Design review of the part built by this model. Coordinates are the model's own, in mm. A direction names the side the tool comes from. Round coordinates to 2 decimals unless told otherwise and drop trailing zeros. Order: outer loops, then holes, each group sorted by start corner. A loop starts at its lowest first (then second) coordinate and runs counter-clockwise, first axis right, second up. Notation, with made-up numbers: (-32, 60) - (15, 60) arc R25 cw to (15, 92) - close; hole circle Ø10 at (75.5, 88). An arc over 180 degrees is marked (long way). Use CSV: the item, a comma, the result in double quotes.
from build123d import *

# Parameters (mm, degrees)
F0_W     = 171.45
F0_H     = 203.2
F0_W_2   = 196.85
F0_H_2   = 228.6
F1_DEPTH = 4.5
F2_DEPTH = 4.5
F3_R     = 6.2865
F4_DEPTH = 2.3
F5_R     = 6.35
F6_DEPTH = 2.3


with BuildPart() as f1:
    # F0 (on Top) → F1 (new body)
    with BuildSketch(Plane.XY):
        Rectangle(F0_W, F0_H)
        Rectangle(F0_W_2, F0_H_2)
        Rectangle(F0_W, F0_H, mode=Mode.SUBTRACT)
    extrude(amount=F1_DEPTH)

    # F0 (on Top) → F2 (cut)
    with BuildSketch(Plane.XY):
        Rectangle(F0_W, F0_H)
    extrude(amount=F2_DEPTH, mode=Mode.SUBTRACT)

    # F3 (on face) → F4 (join)
    with BuildSketch(Plane.XY):
        with Locations((-85.791959, 95.313857)):
            Circle(F3_R)
        with Locations((85.791959, 95.313857)):
            Circle(F3_R)
        with Locations((-85.726304, 82.614026)):
            Circle(F3_R)
        with Locations((-85.660648, 69.914196)):
            Circle(F3_R)
        with Locations((-85.594992, 57.214366)):
            Circle(F3_R)
        with Locations((-85.529336, 44.514535)):
            Circle(F3_R)
        with Locations((-85.463681, 31.814705)):
            Circle(F3_R)
        with Locations((-85.398025, 19.114875)):
            Circle(F3_R)
        with Locations((-85.332369, 6.415045)):
            Circle(F3_R)
        with Locations((-85.266714, -6.284786)):
            Circle(F3_R)
        with Locations((-85.201058, -18.984616)):
            Circle(F3_R)
        with Locations((-85.135402, -31.684446)):
            Circle(F3_R)
        with Locations((-85.069747, -44.384277)):
            Circle(F3_R)
        with Locations((-85.004091, -57.084107)):
            Circle(F3_R)
        with Locations((-84.938435, -69.783937)):
            Circle(F3_R)
        with Locations((-84.87278, -82.483767)):
            Circle(F3_R)
        with Locations((-84.807124, -95.183598)):
            Circle(F3_R)
        with Locations((85.726304, 82.614026)):
            Circle(F3_R)
        with Locations((85.660648, 69.914196)):
            Circle(F3_R)
        with Locations((85.594992, 57.214366)):
            Circle(F3_R)
        with Locations((85.529336, 44.514535)):
            Circle(F3_R)
        with Locations((85.463681, 31.814705)):
            Circle(F3_R)
        with Locations((85.398025, 19.114875)):
            Circle(F3_R)
        with Locations((85.332369, 6.415045)):
            Circle(F3_R)
        with Locations((85.266714, -6.284786)):
            Circle(F3_R)
        with Locations((85.201058, -18.984616)):
            Circle(F3_R)
        with Locations((85.135402, -31.684446)):
            Circle(F3_R)
        with Locations((85.069747, -44.384277)):
            Circle(F3_R)
        with Locations((85.004091, -57.084107)):
            Circle(F3_R)
        with Locations((84.938435, -69.783937)):
            Circle(F3_R)
        with Locations((84.87278, -82.483767)):
            Circle(F3_R)
        with Locations((84.807124, -95.183598)):
            Circle(F3_R)
    extrude(amount=F4_DEPTH)

    # F5 (on face) → F6 (join)
    with BuildSketch(Plane.XY):
        with Locations((-74.604236, 101.599999)):
            Circle(F5_R)
        with Locations((-61.142236, 101.6)):
            Circle(F5_R)
        with Locations((-47.680236, 101.600001)):
            Circle(F5_R)
        with Locations((-34.218236, 101.600003)):
            Circle(F5_R)
        with Locations((-20.756236, 101.600004)):
            Circle(F5_R)
        with Locations((-7.294236, 101.600005)):
            Circle(F5_R)
        with Locations((6.167764, 101.600007)):
            Circle(F5_R)
        with Locations((19.629764, 101.600008)):
            Circle(F5_R)
        with Locations((33.091764, 101.600009)):
            Circle(F5_R)
        with Locations((46.553764, 101.600011)):
            Circle(F5_R)
        with Locations((60.015764, 101.600012)):
            Circle(F5_R)
        with Locations((73.477764, 101.600013)):
            Circle(F5_R)
        with Locations((-74.604236, -101.599999)):
            Circle(F5_R)
        with Locations((-61.142236, -101.6)):
            Circle(F5_R)
        with Locations((-47.680236, -101.600001)):
            Circle(F5_R)
        with Locations((-34.218236, -101.600003)):
            Circle(F5_R)
        with Locations((-20.756236, -101.600004)):
            Circle(F5_R)
        with Locations((-7.294236, -101.600005)):
            Circle(F5_R)
        with Locations((6.167764, -101.600007)):
            Circle(F5_R)
        with Locations((19.629764, -101.600008)):
            Circle(F5_R)
        with Locations((73.477764, -101.600013)):
            Circle(F5_R)
        with Locations((46.553764, -101.600011)):
            Circle(F5_R)
        with Locations((33.091764, -101.600009)):
            Circle(F5_R)
        with Locations((60.015764, -101.600012)):
            Circle(F5_R)
    extrude(amount=F6_DEPTH)


solid = f1.part
1) Insertion check: pin 1 Ø7.5 at (x, y) = (-81, -44.5) entering from +Z; pin 2 Ø5.5 at (x, y) = (83.5, -57) entering from +Z. Each pin has a flat end and moves straight along its axis. Give the tip position at first contact, or say it passes through.
Data:
pin 1,"stops at z = 2.3"
pin 2,"stops at z = 4.5"
2) We need section A-A (x = -35). Give the boundary of the cut face in (y, z).
Data:
outline,"(-114.3, 0) - (-95.3, 0) - (-95.3, 2.3) - (-101.6, 2.3) - (-101.6, 4.5) - (-114.3, 4.5) - close; (95.3, 0) - (114.3, 0) - (114.3, 4.5) - (101.6, 4.5) - (101.6, 2.3) - (95.3, 2.3) - close"
3) To check wall thickness, follow L1, parallel to X at y = -43, z = 3.05 (3 decimals); L2, parallel to Y at x = -64, z = 2.85; L3, parallel to X at y = 7, z = 1.2 (3 decimals). State the ranges of each line that lie inside material, in increasing order. Write a range as from..to.
Data:
L1,"x = -98.425..-85.725, 85.725..98.425"
L2,"y = -114.3..-101.6, 101.6..114.3"
L3,"x = -98.425..-79.073, 79.073..98.425"
4) The part is to be moulded in two halves that separate along Y. For faces 1 (the face through (-61.28, 95.25, 1.13)), 2 (the face through (-88, 9, 4.5)), say which applies: +Y half, -Y half, draft (parallel to the pull), parting line (faces both ways), or undercut.
Data:
face 1,"undercut"
face 2,"draft"
5) For faces 3 (the face through (-20.62, -95.25, 1.13)), 4 (the face through (83, -82, 2.3)), list the 3-axis set-ups (+Z, -Z, +X, -X, +Y, -Y) from which the entire face can be reached by the end or side of a thin tool; tool diameter is ignored.
Data:
face 3,"+Z, -Z"
face 4,"+Z"
6) We need section C-C (z = 1). Give the number of separate pieces and of enclosed holes in the cut face, then the cut area to 3 significant figures.
Data:
separate pieces,"1"
enclosed holes,"2"
area,"13,800 mm2"
7) We need section B-B (y = 81). Give the boundary of the cut face in (x, z) (3 decimals).
Data:
outline,"(-98.425, 0) - (-79.651, 0) - (-79.651, 2.3) - (-85.725, 2.3) - (-85.725, 4.5) - (-98.425, 4.5) - close; (79.651, 0) - (98.425, 0) - (98.425, 4.5) - (85.725, 4.5) - (85.725, 2.3) - (79.651, 2.3) - close"
